Model file for the job. Use its own axes, mm. Face numbers are marked on the shaded views. A direction names the side the tool comes from. Give positions to 0.01 mm unless a question says otherwise; leave off trailing zeros. Write each loop counter-clockwise with the first axis right and the second up, starting at its lowest first coordinate (ties: lowest second). Pieces come first, ordered by that corner, then holes.
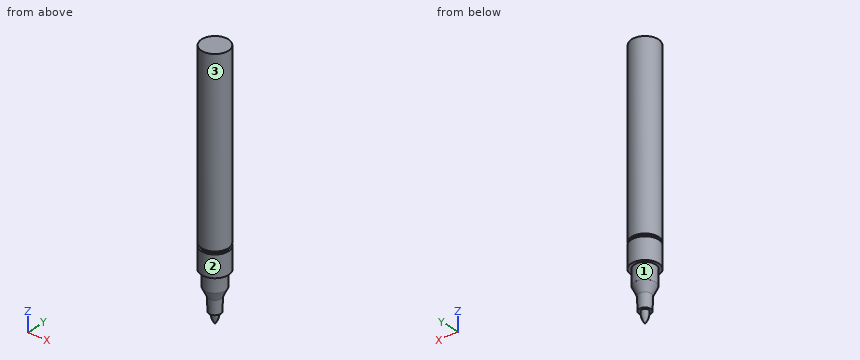
```python
from build123d import *

# Parameters (mm, degrees)
F0_R       = 7.5
F1_DEPTH   = 100
F2_R       = 6.65
F3_DEPTH   = 1.5
F4_R       = 7.615
F5_DEPTH   = 12
F6_R       = 5.95
F8_R       = 5.8
F9_FACE_R  = 5.8
F11_R      = 3.5
F12_FACE_R = 3.5
F14_R      = 3.25


with BuildPart() as f1:
    # F0 (on Top) → F1 (new body)
    with BuildSketch(Plane.XY):
        Circle(F0_R)
    extrude(amount=F1_DEPTH)

    # F2 (on face) → F3 (join)
    with BuildSketch(Plane(origin=(0, 0, 0), x_dir=(1, 0, 0), z_dir=(0, 0, -1))):
        Circle(F2_R)
    extrude(amount=F3_DEPTH)

    # F4 (on face) → F5 (join)
    with BuildSketch(Plane(origin=(0, 0, -1.5), x_dir=(1, 0, 0), z_dir=(0, 0, -1))):
        Circle(F4_R)
    extrude(amount=F5_DEPTH)

    # F6 (on face) → F9 section 0
    with BuildSketch(Plane(origin=(0, 0, -13.5), x_dir=(1, 0, 0), z_dir=(0, 0, -1))):
        Circle(F6_R)
    # F8 (on offset) → F9 section 1
    with BuildSketch(Plane(origin=(0, 0, -22.2), x_dir=(1, 0, 0), z_dir=(0, 0, -1))):
        Circle(F8_R)
    loft()

    # F9_face (on face) → F12 section 0
    with BuildSketch(Plane(origin=(0, 0, -22.2), x_dir=(1, 0, 0), z_dir=(0, 0, -1))):
        Circle(F9_FACE_R)
    # F11 (on offset) → F12 section 1
    with BuildSketch(Plane(origin=(0, 0, -27.2), x_dir=(1, 0, 0), z_dir=(0, 0, -1))):
        Circle(F11_R)
    loft()

    # F12_face (on face) → F15 section 0
    with BuildSketch(Plane(origin=(0, 0, -27.2), x_dir=(1, 0, 0), z_dir=(0, 0, -1))):
        Circle(F12_FACE_R)
    # F14 (on offset) → F15 section 1
    with BuildSketch(Plane(origin=(0, 0, -34.9), x_dir=(1, 0, 0), z_dir=(0, 0, -1))):
        Circle(F14_R)
    loft()

    # F16 (on Right) → F17 (revolve)
    with BuildSketch(Plane.YZ):
        with BuildLine():
            Line((0, -34.9), (-2.05, -34.9))
            ThreePointArc((-2.05, -34.9), (-1.5249883748, -38.2601525263), (0, -41.3))
            Line((0, -41.3), (0, -34.9))
        make_face()
    revolve(axis=Axis((0, 0, -38.1), (0, 0, -1)))


solid = f1.part
```
1. Which spindle directions (+Z, -Z, +X, -X, +Y, -Y) get a long thin tool onto all of the face, cutting with end or side? Do the marked faces 1, 2 and 3. Say none if no direction does.
Calculated:
face 1: -Z
face 2: +Z, -Z
face 3: +Z
2. Pin check, flat tips, straight feed: P1, Ø6, axis at y = 5, z = 48.5, coming from the +X side; P2, Ø5, axis at x = 0, y = 1.5, coming from the -Z side; P3, Ø7.5, axis at x = -3.5, y = 2, coming from the -Z side; P4, Ø5, axis at y = -6, z = 66.5, coming from the +X side. Stop position of each tip, or through.
Calculated:
P1: stops at x = 7.23
P2: stops at z = -41.3
P3: stops at z = -40.89
P4: stops at x = 6.63
3. Probe probe 1 along Z at (x, y) = (3.5, -5.75); probe 2 along X at (y, z) = (-3.5, 41); probe 3 along Z at (x, y) = (-6.25, 0.25). List the from-to ranges inside material, lowest first.
Calculated:
probe 1: z = -13.5 to -1.5, 0 to 100
probe 2: x = -6.63 to 6.63
probe 3: z = -13.5 to 100
4. Slice it at A-A, the plane z = 17.5. Write the cut outline in (x, y), and give its area (3 significant figures).
Calculated:
outline: circle Ø15 at (0, 0)
area: 177 mm2
